Can you work these out from the model? Positions are in its coordinate system, mm. Coordinates: 2 decimals unless noted, no trailing zeros. Order: outer loops, then holes, each group sorted by start corner. A loop starts at its lowest first (then second) coordinate and runs counter-clockwise, first axis right, second up. Notation, with made-up numbers: (8.25, 20) -> (55.25, 20) arc R23 cw to (55.25, 28) -> close; hole circle Ø8 at (65, 22). An arc over 180 degrees is marked (long way). Answer as a JSON object with one key per item and string values. Group by question number.
(1) I need wall thicknesses on line 1 (X direction, y = 45, z = 20); line 2 (Y direction, x = 38.5, z = 743.5); line 3 (Z direction, x = -40, y = -46). Which ranges of each line are inside material? Lowest first, please.
(2) For pin 1 (6 mm diameter, centred on x = 40, z = 20, fed in from -Y); pin 2 (8 mm diameter, centred on y = 0, z = 409, fed in from +X); pin 3 (2 mm diameter, centred on y = 2.5, z = 656, fed in from -X), each with a flat end and sliding along its axis, tell me the tip position at first contact or that it passes through.
(3) I want a section at A-A, the plane x = 18. List the corners of the cut face in (y, z) for me, plus the area to 3 significant figures.
(4) I want a section at C-C, the plane y = 8. List the corners of the cut face in (x, z) for me.
(5) I want a section at B-B, the plane z = 543. List the corners of the cut face in (x, y) for me.
from build123d import *

# Parameters (mm, degrees)
AUFSATZ_LINEAR_AUSTRAGEN1_DEPTH = 890
SKIZZE2_R                       = 3.4
SCHNITT_LINEAR_AUSTRAGEN1_DEPTH = 897.994983264


with BuildPart() as part:
    # Skizze1 → Aufsatz-Linear austragen1 (new body)
    with BuildSketch(Plane.XY):
        Polygon((-50, 50), (50, 50), (50, 40), (5, 40), (5, -40), (50, -40), (50, -50), (-50, -50), (-50, -40), (-5, -40), (-5, 40), (-50, 40), align=None)
    extrude(amount=AUFSATZ_LINEAR_AUSTRAGEN1_DEPTH)

    # Skizze2 → Schnitt-Linear austragen1 (cut, through all)
    with BuildSketch(Plane(origin=(0, 50, 0), x_dir=(1, 0, 0), z_dir=(0, 1, 0))):
        with Locations(Location((40, -870, 0), (0, 0, 270))):
            Circle(SKIZZE2_R)
        with Locations(Location((-40, -870, 0), (0, 0, 180))):
            Circle(SKIZZE2_R)
    schnitt_linear_austragen1 = extrude(amount=-SCHNITT_LINEAR_AUSTRAGEN1_DEPTH, mode=Mode.SUBTRACT)

    # Spiegeln1: Schnitt-Linear austragen1 across plane
    add(schnitt_linear_austragen1.mirror(Plane.XY.offset(445)), mode=Mode.SUBTRACT)


solid = part.part
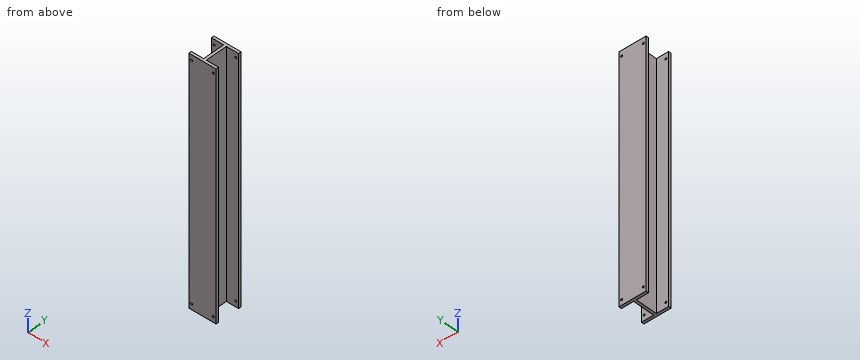
Computed values:
{
 "1": {"line 1": "x = -50 to -43.4, -36.6 to 36.6, 43.4 to 50", "line 2": "y = -50 to -40, 40 to 50", "line 3": "z = 0 to 16.6, 23.4 to 866.6, 873.4 to 890"},
 "2": {"pin 1": "passes through", "pin 2": "stops at x = 5", "pin 3": "stops at x = -5"},
 "3": {"outline": "(-50, 0) -> (-40, 0) -> (-40, 890) -> (-50, 890) -> close; (40, 0) -> (50, 0) -> (50, 890) -> (40, 890) -> close", "area": "17,800 mm2"},
 "4": {"outline": "(-5, 0) -> (5, 0) -> (5, 890) -> (-5, 890) -> close"},
 "5": {"outline": "(-50, -50) -> (50, -50) -> (50, -40) -> (5, -40) -> (5, 40) -> (50, 40) -> (50, 50) -> (-50, 50) -> (-50, 40) -> (-5, 40) -> (-5, -40) -> (-50, -40) -> close"}
}
